For this review, take the finished solid that the model builds, in its own axes (mm). A direction names the side the tool comes from. Round coordinates to 2 decimals unless told otherwise and drop trailing zeros. Loops run counter-clockwise (first coordinate to the right, second up) from the corner with the lowest first, then second, coordinate; pieces in that order, holes last. Notation, with made-up numbers: (-17, 67.25) -> (5, 67.25) arc R20 ccw to (5, 97.25) -> close; hole circle Ø2 at (10.25, 84.25). An arc over 180 degrees is marked (long way). Use one line per item in the form item = value. Start each with the question number.
Autodesk Inventor part; units mm, degrees
ref_plane "core_rod_XY" through (4.5, 0, 0) normal (1, 0, 0) x (0, 0, -1)
ref_plane "core_rod_YZ" through (4.5, 0, 0) normal (0, 0, -1) x (0, 1, 0)
ref_plane "core_rod_ZX" through (4.5, 0, 0) normal (0, 1, 0) x (1, 0, 0)
sketch "Sketch_1" plane through (0, 0, 0) normal (0, 0, 1) x (1, 0, 0)
  line L0 (9.5, 0) -> (0, 0)
  line L1 (0, 0) -> (0, 1.5)
  line L2 (0, 1.5) -> (1, 2.5)
  line L3 (1, 2.5) -> (4.5, 2.5)
  line L4 (4.5, 2.5) -> (4.5, 4)
  line L5 (4.5, 4) -> (9.5, 4)
  line L6 (9.5, 4) -> (9.5, 0)
  line L7 (9.5, 0) -> (0, 0)
revolve "Revolution1" add sketch "Sketch_1" angle 360 about axis through (9.5, 0, 0) along (1, 0, 0)
sketch "Sketch2" plane through (9.5, 0, 0) normal (1, 0, 0) x (0, 0, -1)
  point P0 (0, 0)
hole "Hole1" at (9.5, 0, 0) direction (-1, 0, 0) diameter 2.459 depth 7.7901 tip angle 120 countersink diameter 3.459 countersink angle 90
sketch "Sketch_2" plane through (9.5, 0, 0) normal (1, 0, 0) x (0, 0, -1)
  line L0 (-7, 7) -> (-7, -7)
  line L1 (-7, -7) -> (7, -7)
  line L2 (7, -7) -> (7, 7)
  line L3 (7, 7) -> (-7, 7)
  line L4 (-3.5, 1.9571) -> (-3.5, -1.9571)
  arc A0 (-3.5, -1.9571) -> (3.5, -1.9571) centre (0, 0) ccw
  line L5 (3.5, -1.9571) -> (3.5, 1.9571)
  arc A1 (3.5, 1.9571) -> (-3.5, 1.9571) centre (0, 0) ccw
extrude "Extrusion1" cut sketch "Sketch_2" against normal blind 4
ref_plane "core_rod_XY" through (4.5, 0, 0) normal (1, 0, 0) x (0, 0, -1)
ref_plane "core_rod_YZ" through (4.5, 0, 0) normal (0, 0, -1) x (0, 1, 0)
ref_plane "core_rod_ZX" through (4.5, 0, 0) normal (0, 1, 0) x (1, 0, 0)
properties part number "URLM8_c"
Item 1: Wall thickness on line 1 (Z direction, x = 3.75, y = 0); line 2 (Z direction, x = 4.75, y = 0): over which ranges is each line inside the solid? List them lowest first.
Item 2: For P1, Ø2, axis at y = -1, z = 3, coming from the -X side; P2, Ø1.2, axis at x = 6.5, y = 0, coming from the +Z side; P3, Ø1, axis at y = -1, z = 0.5, coming from the +X side, all flat-tipped, find the tip position at first contact; note any pin that passes through.
Item 3: Take a section at A-A on x = 6. Give the boundary of the cut face in (y, z), plus the area to 3 significant figures.
Item 4: Draft analysis for pull direction Z (two halves, no side actions). For faces 1 (the conical face through (1, 0, 0)), 2 (the flat face through (8, 0, -3.5)), 3 (the cylindrical face through (7.035, 2.15, 3.373)), state which applies: +Z half, -Z half, draft (parallel to the pull), parting line (faces both ways), or undercut.
Item 5: Machinability: for faces 4 (the flat face through (9.5, -2, 0)), 5 (the flat face through (4.5, 2, 2)), 6 (the flat face through (8, 0, 3.5)), 7 (the flat face through (0, 0, 0)), 8 (the cylindrical face through (5.304, 0.748, 0.976)), which of the approach directions +Z, -Z, +X, -X, +Y, -Y give a long, thin tool a straight path to every point of the face, cutting with its end or side? Answer none if there is none.
Item 6: Take a section at B-B on x = 3.5. Give the boundary of the cut face in (y, z).
Item 7: Take a section at C-C on x = 1.5. Give the boundary of the cut face in (y, z).
Results:
q1.line_1 = -2.5 to -1.23, 1.23 to 2.5
q1.line_2 = -4 to -1.23, 1.23 to 4
q2.P1 = 0.66
q2.P2 = 3.5
q2.P3 = 9.39
q3.outline = (-1.94, -3.5) -> (1.94, -3.5) arc R4 ccw to (1.94, 3.5) -> (-1.94, 3.5) arc R4 ccw to start; hole circle Ø2.46 at (0, 0)
q3.area = 42.9 mm2
q4.face_1 = undercut
q4.face_2 = -Z half
q4.face_3 = parting line
q5.face_4 = +Z, -Z, +X, +Y, -Y
q5.face_5 = -X
q5.face_6 = +Z, +X, +Y, -Y
q5.face_7 = +Z, -Z, -X, +Y, -Y
q5.face_8 = +X
q6.outline = circle Ø5 at (0, 0); hole circle Ø2.46 at (0, 0)
q7.outline = circle Ø5 at (0, 0); hole circle Ø1.73 at (0, 0)
